Input: part model. Units: mm. Frame: model coordinates. Face numbers are marked on the shaded views. A direction names the side the tool comes from. Give positions to 0.01 mm unless a question says otherwise; leave off trailing zeros. Order: outer loops, then holes, each group sorted by start corner. A loop starts at its lowest first (then second) coordinate and runs counter-clockwise, first axis right, second up. Notation, with made-up numbers: (-39.5, -21.75) - (-18.5, -21.75) arc R20 cw to (-18.5, -11.75) - close; hole circle Ø3 at (76.25, 11). An arc over 180 degrees is marked (long way). Answer in a Markdown table with one row per item. Add a question column.
1. Section query A-A on y = -5.25. Return loops of the section in (x, z).
2. Contact query for flat-ended pins moving along their axis: pin 1 (10 mm diameter, centred on x = 14, y = 7.5, fed in from +Z); pin 2 (12 mm diameter, centred on x = -15, y = -1, fed in from -Z). Output: stop coordinate, or through.
3. Section query C-C on z = 3.5. Return loops of the section in (x, y).
4. Section query D-D on y = -8. Return loops of the section in (x, z), and give its area (3 significant figures).
5. Access query for the marked faces 1, 2 and 3. Directions: +Z, -Z, +X, -X, +Y, -Y. A direction counts if a zero-diameter tool reaches every point of the face in a straight line with its end or side. Return the directions, or none.
6. Section query B-B on x = 14.5. Return loops of the section in (y, z), and give its area (3 significant figures).
7. Ray query, line 1 (X direction, y = 5.25, z = 1); line 2 (X direction, y = 4, z = 1.5); line 3 (Z direction, x = -18, y = 8). Return the intervals inside material, ascending. Write a range as [from, to].
```python
from build123d import *

# Parameters (mm, degrees)
F0_W         = 40.28548
F0_H         = 20
F0_R         = 1.75
F1_DEPTH     = 10
F3_DEPTH     = 25
F4_R         = 1
F5_T1_DEPTH  = 3.5
F5_S5_W      = 1
F5_S5_H      = 1
F5_T6_DEPTH  = 1
F5_S11_W     = 1
F5_S11_H     = 1
F5_T12_DEPTH = 1
F5_S17_W     = 1
F5_S17_H     = 1
F5_T18_DEPTH = 1
F5_S23_W     = 1
F5_S23_H     = 1
F5_T24_DEPTH = 1


# Not quite as in the source:
# - a fillet or chamfer that OpenCascade refuses, or shapes differently, is made with other operations: its cross-section is extruded or revolved along the edge and cut away or added


with BuildPart() as f1:
    # F0 (on Top) → F1 (new body)
    with BuildSketch(Plane.XY):
        Rectangle(F0_W, F0_H)
        with Locations((-15.39274, -5.25)):
            Circle(F0_R, mode=Mode.SUBTRACT)
        with Locations((15.39274, -5.25)):
            Circle(F0_R, mode=Mode.SUBTRACT)
        with Locations((-15.39274, 5.25)):
            Circle(F0_R, mode=Mode.SUBTRACT)
        with Locations((15.39274, 5.25)):
            Circle(F0_R, mode=Mode.SUBTRACT)
    extrude(amount=F1_DEPTH)

    # F2 (on face) → F3 (cut)
    with BuildSketch(Plane.XZ.offset(10)):
        with BuildLine():
            Line((-4.582575695, 2), (4.582575695, 2))
            ThreePointArc((4.582575695, 2), (0, 5), (-4.582575695, 2))
        make_face()
        with BuildLine():
            Line((-5, 0), (5, 0))
            ThreePointArc((5, 0), (4.8945315647, 1.0215482184), (4.582575695, 2))
            Line((4.582575695, 2), (-4.582575695, 2))
            ThreePointArc((-4.582575695, 2), (-4.8945315647, 1.0215482184), (-5, 0))
        make_face()
        with BuildLine():
            ThreePointArc((-5.6568542495, 2), (0, 6), (5.6568542495, 2))
            Line((5.6568542495, 2), (20.14274, 2))
            Line((20.14274, 2), (20.14274, 10))
            Line((20.14274, 10), (-20.14274, 10))
            Line((-20.14274, 10), (-20.14274, 2))
            Line((-20.14274, 2), (-5.6568542495, 2))
        make_face()
    extrude(amount=-F3_DEPTH, mode=Mode.SUBTRACT)

    # F4
    f4_edges = [f1.edges().sort_by_distance(p)[0] for p in [
        (-20.14274, 0, 2),
        (-12.899797, -10, 2),
        (-12.899797, 10, 2),
        (12.899797, 10, 2),
        (20.14274, 0, 2),
        (12.899797, -10, 2),
    ]]
    fillet(f4_edges, radius=F4_R)

    # F5: fillet of radius 1 on 4 edges, made by hand

    # F5_s2 → F5_t1 (cut)
    with BuildSketch(Plane.XY.offset(-2.5)):
        with BuildLine():
            ThreePointArc((20.14274, -9), (19.8498467812, -9.7071067812), (19.14274, -10))
            Line((19.14274, -10), (20.14274, -10))
            Line((20.14274, -10), (20.14274, -9))
        make_face()
        with BuildLine():
            ThreePointArc((19.14274, 10), (19.8498467812, 9.7071067812), (20.14274, 9))
            Line((20.14274, 9), (20.14274, 10))
            Line((20.14274, 10), (19.14274, 10))
        make_face()
        with BuildLine():
            ThreePointArc((-19.14274, 10), (-19.8498467812, 9.7071067812), (-20.14274, 9))
            Line((-20.14274, 9), (-20.14274, 10))
            Line((-20.14274, 10), (-19.14274, 10))
        make_face()
        with BuildLine():
            ThreePointArc((-20.14274, -9), (-19.8498467812, -9.7071067812), (-19.14274, -10))
            Line((-19.14274, -10), (-20.14274, -10))
            Line((-20.14274, -10), (-20.14274, -9))
        make_face()
    extrude(amount=F5_T1_DEPTH, mode=Mode.SUBTRACT)


with BuildPart() as f5_tool4:
    # F5_s5 → F5_t6 (new body)
    with BuildSketch(Plane.YZ.offset(-19.14274)):
        with Locations((-9.5, 1.5)):
            Rectangle(F5_S5_W, F5_S5_H)
    extrude(amount=-F5_T6_DEPTH)

    # F5_s7 → F5_t8 (revolve, cut)
    with BuildSketch(Plane(origin=(-19.14274, -9, 1), x_dir=(0, 0.7071067812, -0.7071067812), z_dir=(0, 0.7071067812, 0.7071067812))):
        with BuildLine():
            ThreePointArc((0, -1), (1, 0), (0, 1))
            Line((0, 1), (0, -1))
        make_face()
    revolve(axis=Axis((-19.14274, -9, 1), (-1, 0, 0)), mode=Mode.SUBTRACT)


with BuildPart() as f1_1:
    add(f1.part)

    # F5_t3: cut F5_tool4
    add(f5_tool4.part, mode=Mode.SUBTRACT)


with BuildPart() as f5_tool10:
    # F5_s11 → F5_t12 (new body)
    with BuildSketch(Plane.XZ.offset(-9)):
        with Locations((-19.64274, 1.5)):
            Rectangle(F5_S11_W, F5_S11_H)
    extrude(amount=-F5_T12_DEPTH)

    # F5_s13 → F5_t14 (revolve, cut)
    with BuildSketch(Plane(origin=(-19.14274, 9, 1), x_dir=(0.7071067812, 0, -0.7071067812), z_dir=(0.7071067812, 0, 0.7071067812))):
        with BuildLine():
            ThreePointArc((0, -1), (1, 0), (0, 1))
            Line((0, 1), (0, -1))
        make_face()
    revolve(axis=Axis((-19.14274, 9, 1), (0, 1, 0)), mode=Mode.SUBTRACT)


with BuildPart() as f1_2:
    add(f1_1.part)

    # F5_t9: cut F5_tool10
    add(f5_tool10.part, mode=Mode.SUBTRACT)


with BuildPart() as f5_tool16:
    # F5_s17 → F5_t18 (new body)
    with BuildSketch(Plane.XZ.offset(-9)):
        with Locations((19.64274, 1.5)):
            Rectangle(F5_S17_W, F5_S17_H)
    extrude(amount=-F5_T18_DEPTH)

    # F5_s19 → F5_t20 (revolve, cut)
    with BuildSketch(Plane(origin=(19.14274, 9, 1), x_dir=(-0.7071067812, 0, -0.7071067812), z_dir=(0.7071067812, 0, -0.7071067812))):
        with BuildLine():
            ThreePointArc((0, -1), (1, 0), (0, 1))
            Line((0, 1), (0, -1))
        make_face()
    revolve(axis=Axis((19.14274, 9, 1), (0, 1, 0)), mode=Mode.SUBTRACT)


with BuildPart() as f1_3:
    add(f1_2.part)

    # F5_t15: cut F5_tool16
    add(f5_tool16.part, mode=Mode.SUBTRACT)


with BuildPart() as f5_tool22:
    # F5_s23 → F5_t24 (new body)
    with BuildSketch(Plane.YZ.offset(19.14274)):
        with Locations((-9.5, 1.5)):
            Rectangle(F5_S23_W, F5_S23_H)
    extrude(amount=F5_T24_DEPTH)

    # F5_s25 → F5_t26 (revolve, cut)
    with BuildSketch(Plane(origin=(19.14274, -9, 1), x_dir=(0, 0.7071067812, -0.7071067812), z_dir=(0, -0.7071067812, -0.7071067812))):
        with BuildLine():
            ThreePointArc((0, -1), (1, 0), (0, 1))
            Line((0, 1), (0, -1))
        make_face()
    revolve(axis=Axis((19.14274, -9, 1), (1, 0, 0)), mode=Mode.SUBTRACT)


with BuildPart() as f1_4:
    add(f1_3.part)

    # F5_t21: cut F5_tool22
    add(f5_tool22.part, mode=Mode.SUBTRACT)


solid = f1_4.part
```
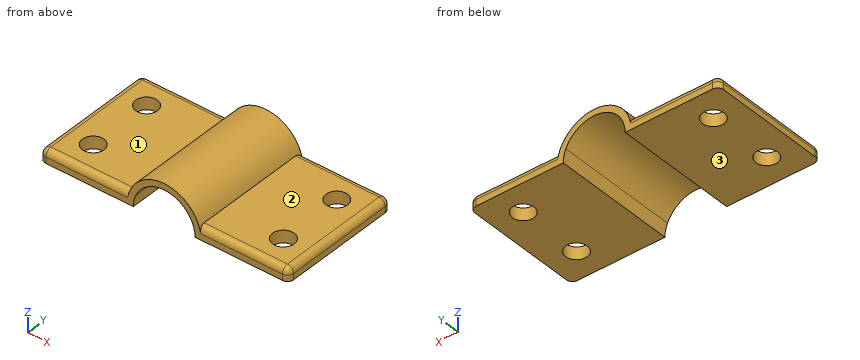
Answer:
| question | item | result |
|---|---|---|
| 1 | outline | (-20.14, 0) - (-17.14, 0) - (-17.14, 2) - (-19.14, 2) arc R1 ccw to (-20.14, 1) - close; (-13.64, 0) - (-5, 0) arc R5 cw to (5, 0) - (13.64, 0) - (13.64, 2) - (5.66, 2) arc R6 ccw to (-5.66, 2) - (-13.64, 2) - close; (17.14, 0) - (20.14, 0) - (20.14, 1) arc R1 ccw to (19.14, 2) - (17.14, 2) - close |
| 2 | pin 1 | stops at z = 2 |
| 2 | pin 2 | stops at z = 0 |
| 3 | outline | (-4.87, -10) - (-3.57, -10) - (-3.57, 10) - (-4.87, 10) - close; (3.57, -10) - (4.87, -10) - (4.87, 10) - (3.57, 10) - close |
| 4 | outline | (-20.14, 0) - (-5, 0) arc R5 cw to (5, 0) - (20.14, 0) - (20.14, 1) arc R1 ccw to (19.14, 2) - (5.66, 2) arc R6 ccw to (-5.66, 2) - (-19.14, 2) arc R1 ccw to (-20.14, 1) - close |
| 4 | area | 73.9 mm² |
| 5 | face 1 | +Z, -X, +Y, -Y |
| 5 | face 2 | +Z, +X, +Y, -Y |
| 5 | face 3 | -Z, +X, -X, +Y, -Y |
| 6 | outline | (-10, 0) - (-6.76, 0) - (-6.76, 2) - (-9, 2) arc R1 ccw to (-10, 1) - close; (-3.74, 0) - (3.74, 0) - (3.74, 2) - (-3.74, 2) - close; (6.76, 0) - (10, 0) - (10, 1) arc R1 ccw to (9, 2) - (6.76, 2) - close |
| 6 | area | 27.5 mm² |
| 7 | line 1 | x = [-20.14, -17.14], [-13.64, -4.9], [4.9, 13.64], [17.14, 20.14] |
| 7 | line 2 | x = [-20.01, -16.62], [-14.17, -4.77], [4.77, 14.17], [16.62, 20.01] |
| 7 | line 3 | z = [0, 2] |
